```python
from build123d import *

# Parameters (mm, degrees)
SKETCH1_W           = 6.35
SKETCH1_H           = 5.08
BOSS_EXTRUDE1_DEPTH = 1.5
SKETCH2_R           = 0.7
SKETCH2_R_2         = 0.45
CUT_EXTRUDE1_DEPTH  = 2.5
CUT_EXTRUDE2_DEPTH  = 0.05
BOSS_EXTRUDE2_DEPTH = 0.01
SKETCH5_W           = 0.05
SKETCH5_H           = 0.6
SKETCH5_W_2         = 0.6
SKETCH5_H_2         = 0.05
CUT_EXTRUDE3_DEPTH  = 2.45
CUT_EXTRUDE4_DEPTH  = 0.05


with BuildPart() as part:
    # Sketch1 → Boss-Extrude1 (new body)
    with BuildSketch(Plane.XY):
        Rectangle(SKETCH1_W, SKETCH1_H)
    extrude(amount=BOSS_EXTRUDE1_DEPTH)

    # Sketch2 → Cut-Extrude1 (cut, through all)
    with BuildSketch(Plane.XY.offset(1.5)):
        with Locations((-3.25, 2.625)):
            Circle(SKETCH2_R)
        with Locations((3.25, 2.625)):
            Circle(SKETCH2_R)
        with Locations((3.25, -2.625)):
            Circle(SKETCH2_R)
        with Locations((-3.25, -2.625)):
            Circle(SKETCH2_R)
        with Locations((0, 2.625)):
            Circle(SKETCH2_R_2)
        with Locations((0, -2.625)):
            Circle(SKETCH2_R_2)
        with Locations((-3.25, 0)):
            Circle(SKETCH2_R_2)
        with Locations((3.25, 0)):
            Circle(SKETCH2_R_2)
    extrude(amount=-CUT_EXTRUDE1_DEPTH, mode=Mode.SUBTRACT)

    # Sketch3 → Cut-Extrude2 (cut)
    with BuildSketch(Plane.XY.offset(1.5)):
        Polygon((-3.175, 1.54), (-2.175, 1.54), (-2.175, 2.54), (-1.575, 2.54), (-1.575, 0.94), (-3.175, 0.94), align=None)
        Polygon((-1.575, -0.94), (-3.175, -0.94), (-3.175, -1.54), (-2.175, -1.54), (-2.175, -2.54), (-1.575, -2.54), align=None)
        Polygon((1.575, -2.54), (1.575, -0.94), (3.175, -0.94), (3.175, -1.54), (2.175, -1.54), (2.175, -2.54), align=None)
        Polygon((1.575, 0.94), (3.175, 0.94), (3.175, 1.54), (2.175, 1.54), (2.175, 2.54), (1.575, 2.54), align=None)
    extrude(amount=-CUT_EXTRUDE2_DEPTH, mode=Mode.SUBTRACT)

    # Sketch4 → Boss-Extrude2 (add)
    with BuildSketch(Plane.XY.offset(1.5)):
        Polygon((-1.495729798, 0.229716512), (0.04659868, 0.955998176), (0.345815845, 0.022984653), (-0.054047094, 0.420127435), align=None)
        Polygon((-0.337060629, 0.894394217), (-0.0051867, 1.050673475), (-0.513753466, 1.364021583), align=None)
        Polygon((0.144089984, 0.962974572), (0.272069208, 0.563912081), (1.164582814, 1.138248631), align=None)
    extrude(amount=BOSS_EXTRUDE2_DEPTH)

    # Sketch5 → Cut-Extrude3 (cut, through all)
    with BuildSketch(Plane.XY.offset(1.45)):
        with Locations((-3.15, 1.24)):
            Rectangle(SKETCH5_W, SKETCH5_H)
        with Locations((-1.875, 2.515)):
            Rectangle(SKETCH5_W_2, SKETCH5_H_2)
        with Locations((1.875, 2.515)):
            Rectangle(SKETCH5_W_2, SKETCH5_H_2)
        with Locations((3.15, 1.24)):
            Rectangle(SKETCH5_W, SKETCH5_H)
        with Locations((3.15, -1.24)):
            Rectangle(SKETCH5_W, SKETCH5_H)
        with Locations((1.875, -2.515)):
            Rectangle(SKETCH5_W_2, SKETCH5_H_2)
        with Locations((-1.875, -2.515)):
            Rectangle(SKETCH5_W_2, SKETCH5_H_2)
        with Locations((-3.15, -1.24)):
            Rectangle(SKETCH5_W, SKETCH5_H)
    extrude(amount=-CUT_EXTRUDE3_DEPTH, mode=Mode.SUBTRACT)

    # Sketch6 → Cut-Extrude4 (cut)
    with BuildSketch(Plane(origin=(0, 0, 0), x_dir=(-1, 0, 0), z_dir=(0, 0, -1))):
        Polygon((3.175, 1.54), (2.175, 1.54), (2.175, 2.54), (1.575, 2.54), (1.575, 0.94), (3.175, 0.94), align=None)
        Polygon((-3.175, 0.94), (-1.575, 0.94), (-1.575, 2.54), (-2.175, 2.54), (-2.175, 1.54), (-3.175, 1.54), align=None)
        Polygon((-1.575, -2.54), (-1.575, -0.94), (-3.175, -0.94), (-3.175, -1.54), (-2.175, -1.54), (-2.175, -2.54), align=None)
        Polygon((1.575, -2.54), (2.175, -2.54), (2.175, -1.54), (3.175, -1.54), (3.175, -0.94), (1.575, -0.94), align=None)
    extrude(amount=-CUT_EXTRUDE4_DEPTH, mode=Mode.SUBTRACT)


solid = part.part
```
Could you check a few things on this model? Use its own coordinates, in mm. Coordinates: 2 decimals unless noted, no trailing zeros. Write each loop counter-clockwise with the first axis right and the second up, starting at its lowest first coordinate (ties: lowest second). Pieces come first, ordered by that corner, then holes. Notation, with made-up numbers: (-31.75, 58) -> (17.25, 58) arc R22 cw to (17.25, 74) -> close; hole circle Ø1 at (86, 80.25). An arc over 180 degrees is marked (long way). One line per question, with ' | ' between items. Start each with the question number.
1. Will this pin go through, and if not, where does the flat tip stop? P1, Ø1.1, axis at x = 3, y = 2, coming from the +Z side.
2. If we section it at B-B (y = 2.25): Please give me the cut outline in (x, z) (3 decimals).
3. If we section it at A-A (y = -1.45): Please give me the cut outline in (x, z) (3 decimals).
4. Please list where these lines run through material, in increasing order: line 1 along Z through (x, y) = (1.5, 0.7); line 2 along Y through (x, z) = (0, 0.35) (3 decimals); line 3 along X through (y, z) = (1.3, 0.6) (3 decimals).
5. Thinking about a two-plate mould opening in X: for faces 1 (the face through (-2.8, 0, 0.8)), 2 (the face through (-2, -2, 1.45)), 3 (the face through (2.6, -1.9, 1.5)), which applies, pulls with the +X half, pulls with the -X half, needs draft (parallel to the pull), parting line crosses it, or undercut?
Return value:
1) P1: stops at z = 1.5
2) outline: (-2.659, 0) -> (-2.175, 0) -> (-2.175, 0.05) -> (-1.575, 0.05) -> (-1.575, 0) -> (-0.249, 0) -> (-0.249, 1.5) -> (-1.575, 1.5) -> (-1.575, 1.45) -> (-2.175, 1.45) -> (-2.175, 1.5) -> (-2.659, 1.5) -> close; (0.249, 0) -> (1.575, 0) -> (1.575, 0.05) -> (2.175, 0.05) -> (2.175, 0) -> (2.659, 0) -> (2.659, 1.5) -> (2.175, 1.5) -> (2.175, 1.45) -> (1.575, 1.45) -> (1.575, 1.5) -> (0.249, 1.5) -> close
3) outline: (-3.125, 0.05) -> (-1.575, 0.05) -> (-1.575, 0) -> (1.575, 0) -> (1.575, 0.05) -> (3.125, 0.05) -> (3.125, 1.45) -> (1.575, 1.45) -> (1.575, 1.5) -> (-1.575, 1.5) -> (-1.575, 1.45) -> (-3.125, 1.45) -> close
4) line 1: z = 0 to 1.5 | line 2: y = -2.175 to 2.175 | line 3: x = -3.125 to 3.125
5) face 1: pulls with the -X half | face 2: undercut | face 3: needs draft
